```python
from build123d import *

# Parameters (mm, degrees)
BOSS_EXTRUDE1_DEPTH = 1.5
BOSS_EXTRUDE2_DEPTH = 13
CUT_EXTRUDE3_DEPTH  = 11.5
FILLET7_R           = 20
FILLET8_R           = 2
SKETCH5_R           = 1.6
CUT_EXTRUDE4_DEPTH  = 5.75


with BuildPart() as part:
    # Sketch1 → Boss-Extrude1 (new body)
    with BuildSketch(Plane.XY):
        Polygon((-4.481783153, -31.006256204), (9.112833652, -37.34553013), (13.762412955, -4.262054337), (-18.076399959, -4.262054337), (-18.076399959, -9.666982278), (-18.076399959, -24.666982278), align=None)
    extrude(amount=BOSS_EXTRUDE1_DEPTH)

    # Sketch2 → Boss-Extrude2 (add)
    with BuildSketch(Plane(origin=(0, 0, 0), x_dir=(-1, 0, 0), z_dir=(0, 0, -1))):
        Polygon((24.076399959, -28.489403843), (24.076399959, -13.489403843), (17.076399959, -13.489403843), (17.076399959, -24.029912017), (7.523455321, -28.48452326), (10.481783153, -34.828677769), align=None)
    extrude(amount=-BOSS_EXTRUDE2_DEPTH)

    # Sketch4 → Cut-Extrude3 (cut)
    with BuildSketch(Plane.XY.offset(13)):
        Polygon((-17.076399959, -13.489403843), (-22.076399959, -13.489403843), (-22.076399959, -27.215263321), (-9.63654663, -33.016062195), (-7.523455321, -28.48452326), (-17.076399959, -24.029912017), align=None)
    extrude(amount=-CUT_EXTRUDE3_DEPTH, mode=Mode.SUBTRACT)

    # Fillet7
    fillet7_edges = [part.edges().sort_by_distance(p)[0] for p in [
        (-24.076399959, -28.489403843, 6.5),
        (-22.076399959, -27.215263321, 7.25),
    ]]
    fillet(fillet7_edges, radius=FILLET7_R)

    # Fillet8
    fillet8_edges = [part.edges().sort_by_distance(p)[0] for p in [
        (-22.076399959, -13.981630974, 1.5),
        (-10.082655912, -32.808038021, 1.5),
        (-18.944228875, -25.219850272, 1.5),
    ]]
    fillet(fillet8_edges, radius=FILLET8_R)

    # Sketch5 → Cut-Extrude4 (cut, symmetric)
    with BuildSketch(Plane(origin=(-22.076399959, 0, 0), x_dir=(0, 0, -1), z_dir=(1, 0, 0))):
        with Locations(Location((-9, -23.189403843, 0), (0, 0, 90))):
            Circle(SKETCH5_R)
    extrude(amount=CUT_EXTRUDE4_DEPTH, both=True, mode=Mode.SUBTRACT)


solid = part.part
```
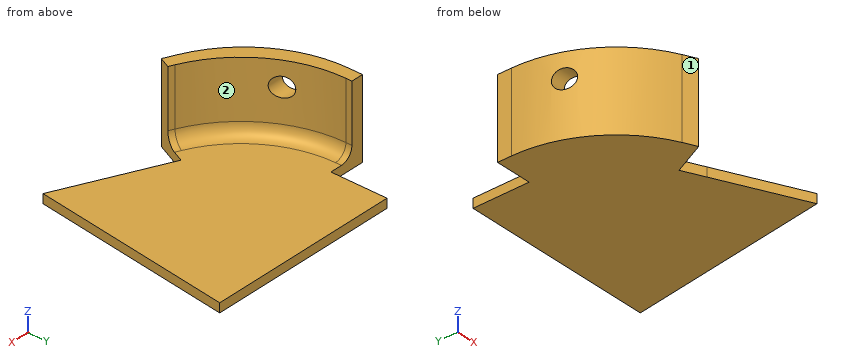
Source: CAD feature listing. Evaluate the final solid. Frame: model axes, mm. Face numbers are marked on the shaded views. A direction names the side the tool comes from. Coordinates: 2 decimals unless noted, no trailing zeros. Write each loop counter-clockwise with the first axis right and the second up, starting at its lowest first coordinate (ties: lowest second). Pieces come first, ordered by that corner, then holes. Notation, with made-up numbers: (18, 33.5) - (39, 33.5) arc R31 cw to (39, 63.5) - close; hole circle Ø4 at (52, 43.5). An arc over 180 degrees is marked (long way). Answer as a JSON object with one key per item and string values.
Q1. First-contact query: pin 1 Ø3.5 at (y, z) = (-23.19, 9) entering from +X; pin 2 Ø6.5 at (x, z) = (-21.5, 9) entering from +Y; pin 3 Ø1 at (y, z) = (-21, 8.5) entering from -X; pin 4 Ø3 at (x, z) = (-6.5, 6.5) entering from -Y. Flat tips, straight axial feed; report the tip coordinate or a pass-through.
Ans:
{"pin 1": "stops at x = -19.12", "pin 2": "stops at y = -13.49", "pin 3": "stops at x = -23.5", "pin 4": "passes through"}
Q2. Section query C-C, the plane y = -8.5. Output: boundary loops of the cut face in (x, z), plus the area to 3 significant figures.
Ans:
{"outline": "(-18.08, 0) - (13.17, 0) - (13.17, 1.5) - (-18.08, 1.5) - close", "area": "46.9 mm2"}
Q3. Section query D-D, the plane x = 6. Output: boundary loops of the cut face in (y, z), plus the area to 3 significant figures.
Ans:
{"outline": "(-35.89, 0) - (-4.26, 0) - (-4.26, 1.5) - (-35.89, 1.5) - close", "area": "47.4 mm2"}
Q4. Section query A-A, the plane z = 6. Output: boundary loops of the cut face in (x, y), plus the area to 3 significant figures.
Ans:
{"outline": "(-24.08, -15.75) arc R20 ccw to (-12.53, -33.87) - (-10.48, -34.83) - (-9.64, -33.02) - (-10.53, -32.6) arc R20 cw to (-22.08, -14.47) - (-22.08, -13.49) - (-24.08, -13.49) - close", "area": "57.5 mm2"}
Q5. Set-up query: the marked faces 1 and 2. Return all of +Z, -Z, +X, -X, +Y, -Y with unobstructed straight access to the full face (end or side cutting, diameter ignored); none if empty.
Ans:
{"face 1": "+Z, -Z, -X, -Y", "face 2": "+Z, +X, +Y"}
Q6. Section query B-B, the plane z = 9. Output: boundary loops of the cut face in (x, y), plus the area to 3 significant figures.
Ans:
{"outline": "(-24.08, -15.75) arc R20 ccw to (-23.2, -21.59) - (-20.77, -21.59) arc R20 cw to (-22.08, -14.47) - (-22.08, -13.49) - (-24.08, -13.49) - close; (-21.92, -24.79) arc R20 ccw to (-12.53, -33.87) - (-10.48, -34.83) - (-9.64, -33.02) - (-10.53, -32.6) arc R20 cw to (-19.21, -24.79) - close", "area": "49.2 mm2"}
Q7. Material intervals for line 1 (Z direction, x = -2.5, y = -23); line 2 (X direction, y = -34, z = 1.25); line 3 (Y direction, x = -20.4, z = 9), sorted ascending. Write a range as [from, to].
Ans:
{"line 1": "z = [0, 1.5]", "line 2": "x = [-12.26, -10.1], [1.94, 9.58]", "line 3": "y = [-27.3, -24.79]"}
